CAD build for the part. Positions are in the model's coordinates, mm. A direction names the side the tool comes from. Give positions to 0.01 mm unless a question says otherwise; leave off trailing zeros. Return JSON: item names as keys, results as strings.
from build123d import *

# Parameters (mm, degrees)
BOSS_EXTRUDE1_DEPTH     = 12.3444
CUT_EXTRUDE1_DEPTH      = 501.459744256
CUT_EXTRUDE1_DEPTH_BACK = 501.459744256
SKETCH12_W              = 6.35
SKETCH12_H              = 25.4
F_1_4_CLEARANCE_HOLE1_D = 6.5278
LPATTERN1_START         = -2.569028042
LPATTERN1_OUTLINE_R     = 3.2639
LPATTERN1_DEPTH         = 12.3444
SKETCH14_W              = 457.208458034
SKETCH14_H              = 25.4
CUT_EXTRUDE2_DEPTH      = 501.552688803


# Read off the part's stored shape, not the designer's step: LPattern1
with BuildPart() as part:
    # Sketch5 for Loft4 → Loft4 section 0
    with BuildSketch(Plane(origin=(0, 203.2, 0), x_dir=(1, 0, 0), z_dir=(0, 1, 0))):
        with BuildLine():
            # circular arc as an exact rational Bezier (weights 1, cos(half-angle), 1)
            Bezier((-50.8, 0), (12.7, 12.200977951), (76.2, 0), weights=[1, 0.982036722, 1])
            Bezier((76.2, 0), (12.7, -12.200977951), (-50.8, 0), weights=[1, 0.982036722, 1])
        make_face()
    # Sketch1 for Loft4 → Loft4 section 1
    with BuildSketch(Plane(origin=(0, 0, 0), x_dir=(1, 0, 0), z_dir=(0, 1, 0))):
        with BuildLine():
            Bezier((0, 0), (228.6, 12.098860838), (457.2, 0), weights=[1, 0.99860236, 1])
            Bezier((457.2, 0), (228.6, -12.098860838), (0, 0), weights=[1, 0.99860236, 1])
        make_face()
    loft()

    # Sketch10 → Boss-Extrude1 (add)
    with BuildSketch(Plane(origin=(-0.017486684, 0, -2.568968528), x_dir=(0, -1, 0), z_dir=(0.006806731520561807, 0, 0.9999768339346702))):
        Polygon((0, 457.189408475), (0, 0), (-25.4, -6.349852895), (-25.4, 409.565511759), align=None)
    extrude(amount=BOSS_EXTRUDE1_DEPTH)

    # Sketch12 → Cut-Extrude1 (cut, two sides: drawn at the far end of the back side and taken through both)
    with BuildSketch(Plane(origin=(0, 0, 0), x_dir=(0.006806731520561809, 0, 0.9999768339346703), z_dir=(-0.9999768339346703, 0, 0.006806731520561809)).offset(-CUT_EXTRUDE1_DEPTH_BACK)):
        with Locations((12.950371958, 12.7)):
            Rectangle(SKETCH12_W, SKETCH12_H)
        with Locations((-5.744028042, 12.7)):
            Rectangle(SKETCH12_W, SKETCH12_H)
    extrude(amount=CUT_EXTRUDE1_DEPTH + CUT_EXTRUDE1_DEPTH_BACK, mode=Mode.SUBTRACT)

    # 1_4 Clearance Hole1 (through all)
    with Locations(Plane(origin=(0.097036893, 0, 14.25568857), x_dir=(0, -1, 0), z_dir=(0.006806731520561807, 0, 0.9999768339346702))):
        with Locations((-12.7, 25.4)):
            Hole(F_1_4_CLEARANCE_HOLE1_D / 2)

    # LPattern1 outline → LPattern1 (cut)
    with BuildSketch(Plane(origin=(0, 0, 0), x_dir=(0.9999768339346702, 0, -0.006806731520561811), z_dir=(0.006806731520561811, 0, 0.9999768339346702)).offset(LPATTERN1_START)):
        with Locations((76.198823164, 12.7)):
            Circle(LPATTERN1_OUTLINE_R)
        with Locations((126.997646328, 12.7)):
            Circle(LPATTERN1_OUTLINE_R)
        with Locations((177.796469492, 12.7)):
            Circle(LPATTERN1_OUTLINE_R)
        with Locations((228.595292656, 12.7)):
            Circle(LPATTERN1_OUTLINE_R)
        with Locations((279.394115819, 12.7)):
            Circle(LPATTERN1_OUTLINE_R)
        with Locations((330.192938983, 12.7)):
            Circle(LPATTERN1_OUTLINE_R)
        with Locations((380.991762147, 12.7)):
            Circle(LPATTERN1_OUTLINE_R)
    extrude(amount=LPATTERN1_DEPTH, mode=Mode.SUBTRACT)

    # Sketch14 → Cut-Extrude2 (cut, through all)
    with BuildSketch(Plane(origin=(0.066538332, 0, 9.775145501), x_dir=(0.9999768339346702, 0, -0.006806731520561792), z_dir=(0.006806731520561792, 0, 0.9999768339346703))):
        with Locations((228.585179458, -12.6238)):
            Rectangle(SKETCH14_W, SKETCH14_H)
    extrude(amount=-CUT_EXTRUDE2_DEPTH, mode=Mode.SUBTRACT)


solid = part.part
1. Drop flat-ended pins along their axis: P1, Ø8, axis at x = 219.5, y = 96, coming from the +Z side; P2, Ø6, axis at x = 71, y = 84, coming from the -Z side. Give the stop position or say it passes through.
Values follow:
{"P1": "stops at z = 4.09", "P2": "stops at z = -5.06"}
2. Which spindle directions (+Z, -Z, +X, -X, +Y, -Y) get a long thin tool onto all of the face, cutting with end or side? Do faces 1 (the face through (225, 0.076, 2)), 2 (the face through (153, 25.4, 6)). Say none if no direction does.
Values follow:
{"face 1": "+Z, -Z, +X, -X, -Y", "face 2": "+Z"}
3. Drill centre lines: probe 1 along Z at (x, y) = (418.5, 13.5); probe 2 along Y at (x, z) = (47.5, 9); probe 3 along Z at (x, y) = (86, 143). Where is each one in solid material? Low to high.
Values follow:
{"probe 1": "z = -5.42 to 6.93", "probe 2": "y = 0.08 to 25.4", "probe 3": "z = -6 to 6"}
